```python
from build123d import *

# Parameters (mm, degrees)
OUTER_CUT_DEPTH   = 1.4986
SLOTS_DEPTH       = 192.473590105
SKETCH3_R         = 1.5875
MOUNT_HOLES_DEPTH = 192.473590105


with BuildPart() as part:
    # Sketch1 → Outer Cut (new, symmetric)
    with BuildSketch(Plane(origin=(0, 0, 0), x_dir=(0, 0, -1), z_dir=(1, 0, 0))):
        with BuildLine():
            Line((-184.15, -19.05), (184.15, -19.05))
            ThreePointArc((184.15, -19.05), (188.640128061, -17.190128061), (190.5, -12.7))
            Line((190.5, -12.7), (190.5, 12.7))
            ThreePointArc((190.5, 12.7), (188.640128061, 17.190128061), (184.15, 19.05))
            Line((184.15, 19.05), (-184.15, 19.05))
            ThreePointArc((-184.15, 19.05), (-188.640128061, 17.190128061), (-190.5, 12.7))
            Line((-190.5, 12.7), (-190.5, -12.7))
            ThreePointArc((-190.5, -12.7), (-188.640128061, -17.190128061), (-184.15, -19.05))
        make_face()
    extrude(amount=OUTER_CUT_DEPTH, both=True)

    # Sketch2 → Slots (cut, through all)
    with BuildSketch(Plane(origin=(1.4986, 0, 0), x_dir=(0, 0, -1), z_dir=(1, 0, 0))):
        with BuildLine():
            Line((-177.8, 3.175), (177.8, 3.175))
            ThreePointArc((177.8, 3.175), (180.975, 0), (177.8, -3.175))
            Line((177.8, -3.175), (-177.8, -3.175))
            ThreePointArc((-177.8, -3.175), (-180.975, 0), (-177.8, 3.175))
        make_face()
    extrude(amount=-SLOTS_DEPTH, mode=Mode.SUBTRACT)

    # Sketch3 → Mount Holes (cut, through all)
    with BuildSketch(Plane(origin=(1.4986, 0, 0), x_dir=(0, 0, -1), z_dir=(1, 0, 0))):
        with Locations((-184.15, 12.7)):
            Circle(SKETCH3_R)
        with Locations((-174.625, 12.7)):
            Circle(SKETCH3_R)
        with Locations((-174.625, -12.7)):
            Circle(SKETCH3_R)
        with Locations((-184.15, -12.7)):
            Circle(SKETCH3_R)
        with Locations((174.625, 12.7)):
            Circle(SKETCH3_R)
        with Locations((184.15, 12.7)):
            Circle(SKETCH3_R)
        with Locations((184.15, -12.7)):
            Circle(SKETCH3_R)
        with Locations((174.625, -12.7)):
            Circle(SKETCH3_R)
    extrude(amount=-MOUNT_HOLES_DEPTH, mode=Mode.SUBTRACT)


solid = part.part
```
Geometry: final body of the model. Coordinates: model frame, mm. Coordinates: 2 decimals unless noted, no trailing zeros. Write each loop counter-clockwise with the first axis right and the second up, starting at its lowest first coordinate (ties: lowest second). Pieces come first, ordered by that corner, then holes. Notation, with made-up numbers: M 79.25,85.5 L 104.25,85.5 A12 ccw 104.25,101.5 Z; hole C -27,34 d7. An arc over 180 degrees is marked long. Answer as CSV lines item,"result". Start each with the question number.
Q1. Cut plane B-B on x = 0.15. Count the separate pieces of the cut face and the enclosed holes in it, then the cut area to 3 significant figures.
Q2. Cut plane C-C on y = 0. Return the cut outline in (x, z) (3 decimals), then the cut area to 3 significant figures.
Q3. Line query: line 1 (Y direction, x = 0.2, z = -184.15); line 2 (Y direction, x = -0.65, z = 173) (3 decimals); line 3 (Z direction, x = -0.35, y = 14). Output: solid intervals per line, ascending. Write a range as from..to.
Q4. Pin query (flat end, axial travel): P1, Ø2.5, axis at y = 12.7, z = 174.625, coming from the +X side; P2, Ø4, axis at y = -12.7, z = -184.15, coming from the +X side. Return the tip coordinate at first contact, or that it passes through.
Q5. Cut plane A-A on z = -43.5. Return the cut outline in (x, y) (3 decimals), then the cut area to 3 significant figures.
Findings below:
1,separate pieces,"1"
1,enclosed holes,"9"
1,area,"12,100 mm2"
2,outline,"M -1.499,-190.5 L 1.499,-190.5 L 1.499,-180.975 L -1.499,-180.975 Z; M -1.499,180.975 L 1.499,180.975 L 1.499,190.5 L -1.499,190.5 Z"
2,area,"57.1 mm2"
3,line 1,"y = -19.05..-14.29, -11.11..11.11, 14.29..19.05"
3,line 2,"y = -19.05..-3.175, 3.175..19.05"
3,line 3,"z = -190.37..-185.06, -183.24..-175.54, -173.71..173.71, 175.54..183.24, 185.06..190.37"
4,P1,"passes through"
4,P2,"stops at x = 1.5"
5,outline,"M -1.499,-19.05 L 1.499,-19.05 L 1.499,-3.175 L -1.499,-3.175 Z; M -1.499,3.175 L 1.499,3.175 L 1.499,19.05 L -1.499,19.05 Z"
5,area,"95.2 mm2"
